Read the model definition and answer for the solid it produces. Units are mm, in the model's axes. Coordinates: 2 decimals unless noted, no trailing zeros. Order: outer loops, then holes, each group sorted by start corner. A loop starts at its lowest first (then second) coordinate and runs counter-clockwise, first axis right, second up.
```python
from build123d import *

# Parameters (mm, degrees)
SKETCH1_W           = 146
SKETCH1_H           = 161
BOSS_EXTRUDE1_DEPTH = 3
SKETCH2_W           = 26
SKETCH2_H           = 3
SKETCH2_W_2         = 3
SKETCH2_H_2         = 30
SKETCH2_W_3         = 60
SKETCH2_H_3         = 25
CUT_EXTRUDE1_DEPTH  = 3
SKETCH3_W           = 146
SKETCH3_H           = 62.32
CUT_EXTRUDE2_DEPTH  = 10
SKETCH4_R           = 1.6
CUT_EXTRUDE3_DEPTH  = 10


with BuildPart() as part:
    # Sketch1 → Boss-Extrude1 (new body)
    with BuildSketch(Plane(origin=(0, 0, 0), x_dir=(1, 0, 0), z_dir=(0, 1, 0))):
        Rectangle(SKETCH1_W, SKETCH1_H)
    extrude(amount=BOSS_EXTRUDE1_DEPTH)

    # Sketch2 → Cut-Extrude1 (cut)
    with BuildSketch(Plane(origin=(0, 3, 0), x_dir=(1, 0, 0), z_dir=(0, 1, 0))):
        with Locations((0, 79)):
            Rectangle(SKETCH2_W, SKETCH2_H)
        with Locations((-71.5, 15.5)):
            Rectangle(SKETCH2_W_2, SKETCH2_H_2)
        Polygon((-73, 80.5), (-73, 60.5), (-70, 60.5), (-70, 77.5), (-43, 77.5), (-43, 80.5), align=None)
        Polygon((73, 80.5), (73, 60.5), (70, 60.5), (70, 77.5), (43, 77.5), (43, 80.5), align=None)
        with Locations((71.5, 15.5)):
            Rectangle(SKETCH2_W_2, SKETCH2_H_2)
        with Locations((-71.5, -44.5)):
            Rectangle(SKETCH2_W_2, SKETCH2_H_2)
        Polygon((-70, -79.5), (-73, -79.5), (-73, -80.5), (-43, -80.5), (-43, -77.5), (-70, -77.5), align=None)
        with Locations((71.5, -44.5)):
            Rectangle(SKETCH2_W_2, SKETCH2_H_2)
        Polygon((70, -79.5), (73, -79.5), (73, -80.5), (70, -80.5), (43, -80.5), (43, -77.5), (70, -77.5), align=None)
        with Locations((0, -79)):
            Rectangle(SKETCH2_W, SKETCH2_H)
        with Locations((17, 60)):
            Rectangle(SKETCH2_W_3, SKETCH2_H_3)
    extrude(amount=-CUT_EXTRUDE1_DEPTH, mode=Mode.SUBTRACT)

    # Sketch3 → Cut-Extrude2 (cut)
    with BuildSketch(Plane(origin=(0, 0, 0), x_dir=(-1, 0, 0), z_dir=(0, -1, 0))):
        with Locations((0, -49.34)):
            Rectangle(SKETCH3_W, SKETCH3_H)
    extrude(amount=-CUT_EXTRUDE2_DEPTH, mode=Mode.SUBTRACT)

    # Sketch4 → Cut-Extrude3 (cut)
    with BuildSketch(Plane.XZ):
        with Locations(Location((62.25, -33.75, 0), (0, 0, 270))):
            Circle(SKETCH4_R)
        with Locations(Location((-65, -23.3, 0), (0, 0, 270))):
            Circle(SKETCH4_R)
    extrude(amount=-CUT_EXTRUDE3_DEPTH, mode=Mode.SUBTRACT)


solid = part.part
```
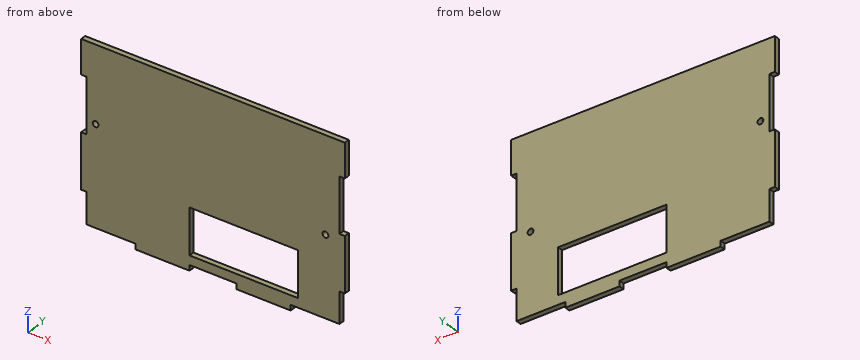
1) A cutting plane is placed at B-B, the plane x = -65. Determine the outline of the cut face in (y, z).
A:
outline: (0, -77.5) - (3, -77.5) - (3, -24.9) - (0, -24.9) - close; (0, -21.7) - (3, -21.7) - (3, 18.18) - (0, 18.18) - close
2) A cutting plane is placed at D-D, the plane x = 54. Determine the outline of the cut face in (y, z).
A:
outline: (0, -77.5) - (3, -77.5) - (3, 18.18) - (0, 18.18) - close
3) Straight lines are drawn through the part: line 1 (X direction, y = 2.1, z = -53); line 2 (Z direction, x = -10.5, y = 2.05); line 3 (Z direction, x = 19, y = 1.5). For each, find the intervals that lie inside material, in ascending order.
A:
line 1: x = -73 to -13, 47 to 73
line 2: z = -77.5 to -72.5, -47.5 to 18.18
line 3: z = -80.5 to -72.5, -47.5 to 18.18
4) A cutting plane is placed at C-C, the plane y = 1.5. State how many separate pieces and enclosed holes the cut face has, and give its area (3 significant figures).
A:
separate pieces: 1
enclosed holes: 3
area: 12,400 mm2
5) A cutting plane is placed at A-A, the plane z = -70. Determine the outline of the cut face in (x, y), and give its area (3 significant figures).
A:
outline: (-70, 0) - (-13, 0) - (-13, 3) - (-70, 3) - close; (47, 0) - (70, 0) - (70, 3) - (47, 3) - close
area: 240 mm2
6) Flat-ended cylindrical pins translate along their axes: pin 1 Ø0.9 at (x, y) = (71, 1) entering from -Z; pin 2 Ø0.9 at (y, z) = (2, -72) entering from +X; pin 3 Ø1.5 at (y, z) = (1, -78.5) entering from -X. Find the tip coordinate at first contact, or state that the pin passes through.
A:
pin 1: stops at z = -60.5
pin 2: stops at x = 70
pin 3: stops at x = -43
